Model file for the job. Use its own axes, mm. Face numbers are marked on the shaded views. A direction names the side the tool comes from. Round coordinates to 2 decimals unless told otherwise and drop trailing zeros. Write each loop counter-clockwise with the first axis right and the second up, starting at its lowest first coordinate (ties: lowest second). Pieces come first, ordered by that corner, then holes. Notation, with made-up numbers: (13.5, -2.75) - (61.5, -2.75) arc R18 cw to (61.5, 30.25) - close; hole circle Ø6 at (-9.75, -26.5). An arc over 180 degrees is marked (long way). One line per item, written item: value.
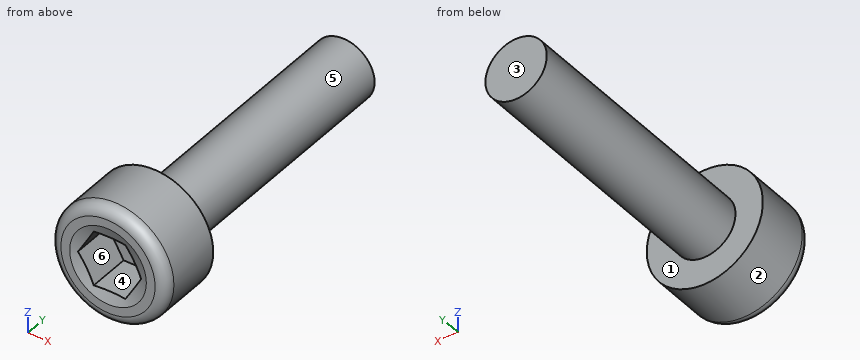
from build123d import *

# Parameters (mm, degrees)
CUT_EXTRUDE1_DEPTH = 2
FILLET1_R          = 0.5


with BuildPart() as part:
    # Sketch2 → Revolve1 (revolve)
    with BuildSketch(Plane.XY):
        Polygon((0, 0), (2.65, 0), (2.65, 3), (1.4, 3), (1.4, 15), (0, 15), align=None)
    revolve(axis=Axis((0, 0, 0), (0, 1, 0)))

    # Sketch3 → Cut-Extrude1 (cut)
    with BuildSketch(Plane.XZ):
        Polygon((-1.443375673, 0), (-0.721687836, -1.25), (0.721687836, -1.25), (1.443375673, 0), (0.721687836, 1.25), (-0.721687836, 1.25), align=None)
    extrude(amount=-CUT_EXTRUDE1_DEPTH, mode=Mode.SUBTRACT)

    # Sketch6 → Cut-Revolve1 (revolve, cut)
    with BuildSketch(Plane(origin=(0, 0, 0), x_dir=(-1, 0, 0), z_dir=(0, 0, -1))):
        with BuildLine():
            Line((0, 0), (0, 0.3))
            ThreePointArc((0, 0.3), (-0.887764045, 0.22445693), (-1.75, 0))
            Line((-1.75, 0), (0, 0))
        make_face()
    revolve(axis=Axis((0, 0, 0), (0, 1, 0)), mode=Mode.SUBTRACT)

    # Fillet1
    fillet1_edges = [part.edges().sort_by_distance(p)[0] for p in [
        (-2.65, 0, 0),
    ]]
    fillet(fillet1_edges, radius=FILLET1_R)


solid = part.part
1. Drop flat-ended pins along their axis: pin 1 (1.2 mm diameter, centred on x = 0, z = -0.5, fed in from -Y); pin 2 (1 mm diameter, centred on x = 1, y = 10.5, fed in from +Z); pin 3 (1 mm diameter, centred on x = -1.5, z = -2, fed in from +Y). Give the stop position or say it passes through.
Report:
pin 1: y = 2
pin 2: z = 1.31
pin 3: y = 3
2. Tool access for the marked faces 1 and 2: list every direction of +Z, -Z, +X, -X, +Y, -Y with a clear straight run to the whole face (end or side of a thin tool).
Report:
face 1: +Y
face 2: +Y, -Y
3. Wall check: probe 1 along Y at (x, z) = (0.1, -0.05); probe 2 along Y at (x, z) = (1.9, -0.25); probe 3 along Z at (x, y) = (0, 11.75). Give the ranges that are in metal, low to high. Write a range as [from, to].
Report:
probe 1: [2, 15]
probe 2: [0, 3]
probe 3: [-1.4, 1.4]
4. Band-saw the part on A-A on x = 0. Write the cut outline in (y, z), plus the area to 3 significant figures.
Report:
outline: (0, -2.15) arc R0.5 ccw to (0.5, -2.65) - (3, -2.65) - (3, -1.4) - (15, -1.4) - (15, 1.4) - (3, 1.4) - (3, 2.65) - (0.5, 2.65) arc R0.5 ccw to (0, 2.15) - (0, 1.75) arc R5.25 cw to (0.15, 1.25) - (2, 1.25) - (2, -1.25) - (0.15, -1.25) arc R5.25 cw to (0, -1.75) - close
area: 44.3 mm²
5. Mould opens along Z. For the marked faces 3, 4, 5 and 6 say: released by +Z, released by -Z, zero draft, split by the parting line, or undercut.
Report:
face 3: zero draft
face 4: undercut
face 5: split by the parting line
face 6: undercut
6. Band-saw the part on B-B on y = 12.75. Write the cut outline in (x, z).
Report:
outline: circle Ø2.8 at (0, 0)
